Input: part model. Units: mm. Frame: model coordinates. A direction names the side the tool comes from. Give positions to 0.01 mm unless a question says otherwise; leave off trailing zeros. Write each loop counter-clockwise with the first axis right and the second up, starting at its lowest first coordinate (ties: lowest second). Pieces come first, ordered by that corner, then holes. Notation, with made-up numbers: (57.5, -22.5) - (65.5, -22.5) arc R17 ccw to (65.5, -10.5) - close; hole circle Ø1 at (70, 13.25). An arc over 180 degrees is marked (long way). Answer as CSV lines item,"result". Start each with the question number.
from build123d import *

# Parameters (mm, degrees)
F0_R     = 1.5875
F1_DEPTH = 70


with BuildPart() as f1:
    # F0 (on Top) → F1 (new body)
    with BuildSketch(Plane.XY):
        with BuildLine():
            ThreePointArc((42.5527261375, -14.32743865), (44.3092958846, -7.2592215983), (44.9, 0))
            ThreePointArc((44.9, 0), (34.7433650607, 28.4413182581), (8.8684372267, 44.0154611603))
            ThreePointArc((8.8684372267, 44.0154611603), (9.8318086389, 41.6194720159), (10.16, 39.058))
            ThreePointArc((10.16, 39.058), (9.9243037361, 36.8822713051), (9.2281505209, 34.807489682))
            ThreePointArc((9.2281505209, 34.807489682), (28.53967239, 21.9592167408), (36.01, 0))
            ThreePointArc((36.01, 0), (35.6956896759, -4.7474033498), (34.758245567, -9.4119320599))
            ThreePointArc((34.758245567, -9.4119320599), (39.2448159004, -10.9351892811), (42.5527261375, -14.32743865))
        make_face()
        with BuildLine():
            ThreePointArc((10.16, 39.058), (9.8318086389, 41.6194720159), (8.8684372267, 44.0154611603))
            ThreePointArc((8.8684372267, 44.0154611603), (0, 44.9), (-8.8684372267, 44.0154611603))
            ThreePointArc((-8.8684372267, 44.0154611603), (-10.1522562376, 39.4546021771), (-9.2281505209, 34.807489682))
            ThreePointArc((-9.2281505209, 34.807489682), (0, 36.01), (9.2281505209, 34.807489682))
            ThreePointArc((9.2281505209, 34.807489682), (9.9243037361, 36.8822713051), (10.16, 39.058))
        make_face()
        with Locations((0, 39.058)):
            Circle(F0_R, mode=Mode.SUBTRACT)
        with BuildLine():
            ThreePointArc((33.6842889108, -29.6880225103), (38.8845406299, -22.45), (42.5527261375, -14.32743865))
            ThreePointArc((42.5527261375, -14.32743865), (39.2448159004, -10.9351892811), (34.758245567, -9.4119320599))
            ThreePointArc((34.758245567, -9.4119320599), (31.1855747903, -18.005), (25.5300950461, -25.3955576221))
            ThreePointArc((25.5300950461, -25.3955576221), (29.0925596628, -28.519412896), (33.6842889108, -29.6880225103))
        make_face()
        with Locations((33.825220221, -19.529)):
            Circle(F0_R, mode=Mode.SUBTRACT)
        with BuildLine():
            ThreePointArc((-9.2281505209, 34.807489682), (-10.1522562376, 39.4546021771), (-8.8684372267, 44.0154611603))
            ThreePointArc((-8.8684372267, 44.0154611603), (-38.8845406299, 22.45), (-42.5527261375, -14.32743865))
            ThreePointArc((-42.5527261375, -14.32743865), (-39.2448159004, -10.9351892811), (-34.758245567, -9.4119320599))
            ThreePointArc((-34.758245567, -9.4119320599), (-31.1855747903, 18.005), (-9.2281505209, 34.807489682))
        make_face()
        with BuildLine():
            ThreePointArc((-33.6842889108, -29.6880225103), (0, -44.9), (33.6842889108, -29.6880225103))
            ThreePointArc((33.6842889108, -29.6880225103), (29.0925596628, -28.519412896), (25.5300950461, -25.3955576221))
            ThreePointArc((25.5300950461, -25.3955576221), (0, -36.01), (-25.5300950461, -25.3955576221))
            ThreePointArc((-25.5300950461, -25.3955576221), (-29.0925596628, -28.519412896), (-33.6842889108, -29.6880225103))
        make_face()
        with BuildLine():
            ThreePointArc((25.5300950461, -25.3955576221), (31.1855747903, -18.005), (34.758245567, -9.4119320599))
            ThreePointArc((34.758245567, -9.4119320599), (25.0264021186, -14.449), (25.5300950461, -25.3955576221))
        make_face()
        with BuildLine():
            ThreePointArc((-34.758245567, -9.4119320599), (-39.2448159004, -10.9351892811), (-42.5527261375, -14.32743865))
            ThreePointArc((-42.5527261375, -14.32743865), (-38.8845406299, -22.45), (-33.6842889108, -29.6880225103))
            ThreePointArc((-33.6842889108, -29.6880225103), (-29.0925596628, -28.519412896), (-25.5300950461, -25.3955576221))
            ThreePointArc((-25.5300950461, -25.3955576221), (-31.1855747903, -18.005), (-34.758245567, -9.4119320599))
        make_face()
        with Locations((-33.825220221, -19.529)):
            Circle(F0_R, mode=Mode.SUBTRACT)
        with BuildLine():
            ThreePointArc((9.2281505209, 34.807489682), (0, 36.01), (-9.2281505209, 34.807489682))
            ThreePointArc((-9.2281505209, 34.807489682), (0, 28.898), (9.2281505209, 34.807489682))
        make_face()
        with BuildLine():
            ThreePointArc((-23.665220221, -19.529), (-26.9788320315, -12.0221651971), (-34.758245567, -9.4119320599))
            ThreePointArc((-34.758245567, -9.4119320599), (-31.1855747903, -18.005), (-25.5300950461, -25.3955576221))
            ThreePointArc((-25.5300950461, -25.3955576221), (-24.1426567232, -22.6069155465), (-23.665220221, -19.529))
        make_face()
    extrude(amount=F1_DEPTH)


solid = f1.part
1) Pull-direction query (Y, two-part tool) for faces 1 (the flat face through (-27, -16, 70)), 2 (the cylindrical face through (0.397, -36.008, 34.51)); classes: +Y half, -Y half, draft (parallel to the pull), parting line (faces both ways), or undercut.
2) Cut plane C-C on y = 14. Output: boundary loops of the cut face in (x, z), and give its area (3 significant figures).
3) Contact query for flat-ended pins moving along their axis: P1, Ø3, axis at y = -13.5, z = 19.5, coming from the +X side; P2, Ø8, axis at x = 20.5, z = 11, coming from the +Y side; P3, Ø8, axis at x = 12, z = 47.5, coming from the -Y side. Output: stop coordinate, or through.
4) Reachability of faces 3 (the cylindrical face through (25.11, -14.31, 34.51)), 4 (the flat face through (-27, -16, 0)) from +Z, -Z, +X, -X, +Y, -Y: full face, straight path, thin tool, end or side. Return the list, or none.
5) Cut plane B-B on z = 56. Output: boundary loops of the cut face in (x, y) (1 decimal).
6) Cut plane A-A on x = 0. Output: boundary loops of the cut face in (y, z), and give its area (3 significant figures).
7) Material intervals for line 1 (X direction, y = -18.5, z = 25); line 2 (Y direction, x = -16.5, z = 3); line 3 (X direction, y = 26, z = 66.5), sorted ascending. Write a range as from..to.
8) Cut plane D-D on x = 12. Output: boundary loops of the cut face in (y, z), and give its area (3 significant figures).
Numbers:
1,face 1,"draft"
1,face 2,"undercut"
2,outline,"(-42.66, 0) - (-33.18, 0) - (-33.18, 70) - (-42.66, 70) - close; (33.18, 0) - (42.66, 0) - (42.66, 70) - (33.18, 70) - close"
2,area,"1,330 mm²"
3,P1,"stops at x = 43.27"
3,P2,"stops at y = 41.76"
3,P3,"stops at y = -44.18"
4,face 3,"+Z, -Z"
4,face 4,"-Z, +X, -X, +Y, -Y"
5,outline,"circle Ø89.8 at (0, 0); hole circle Ø3.2 at (-33.8, -19.5); hole (-34.8, -9.4) arc R10.2 cw to (-25.5, -25.4) arc R36 ccw to (25.5, -25.4) arc R10.2 cw to (34.8, -9.4) arc R36 ccw to (9.2, 34.8) arc R10.2 cw to (-9.2, 34.8) arc R36 ccw to start; hole circle Ø3.2 at (0, 39.1); hole circle Ø3.2 at (33.8, -19.5)"
6,outline,"(-44.9, 0) - (-36.01, 0) - (-36.01, 70) - (-44.9, 70) - close; (28.9, 0) - (37.47, 0) - (37.47, 70) - (28.9, 70) - close; (40.65, 0) - (44.9, 0) - (44.9, 70) - (40.65, 70) - close"
6,area,"1,520 mm²"
7,line 1,"x = -40.91..-35.03, -32.62..-23.72, 23.72..32.62, 35.03..40.91"
7,line 2,"y = -41.76..-32.01, 32.01..41.76"
7,line 3,"x = -36.61..-24.91, 24.91..36.61"
8,outline,"(-43.27, 0) - (-33.95, 0) - (-33.95, 70) - (-43.27, 70) - close; (33.95, 0) - (43.27, 0) - (43.27, 70) - (33.95, 70) - close"
8,area,"1,300 mm²"
